Geometry: final body of the model. Coordinates: model frame, mm. Face numbers are marked on the shaded views. Give positions to 0.01 mm unless a question says otherwise; leave off trailing zeros. Write each loop counter-clockwise with the first axis right and the second up, starting at its lowest first coordinate (ties: lowest second). Pieces come first, ordered by that corner, then holes. Notation, with made-up numbers: (70, 87.5) - (126, 87.5) arc R13 ccw to (126, 92.5) - close; hole circle Ø2 at (28.5, 85). An arc over 180 degrees is marked (long way). Use CSV: the item, a comma, the result in double quotes. Start each with the question number.
(1) Section A-A on x = 0. Output: boundary loops of the cut face in (y, z), and give its area (3 significant figures).
(2) Section D-D on z = -3.5. Output: boundary loops of the cut face in (x, y), and give its area (3 significant figures).
(3) Line query: probe 1 along Z at (x, y) = (-21, -23); probe 2 along X at (y, z) = (22, 24.5) (3 decimals); probe 3 along Z at (x, y) = (20.25, 22.75) (3 decimals). Output: solid intervals per line, ascending. Write a range as [from, to].
(4) Section B-B on y = -12. Output: boundary loops of the cut face in (x, z).
(5) Draft query along Y for the marked faces 1, 2 and 3. Return one class per face: released by +Y, released by -Y, zero draft, split by the parting line, or undercut.
(6) First-contact query: pin 1 Ø10 at (x, y) = (9, 6) entering from -Z; pin 2 Ø2.5 at (x, z) = (20.25, -24.5) entering from -Y; pin 3 Ø1.8 at (x, z) = (-20.25, 24.5) entering from +Y; pin 4 Ø5 at (x, y) = (0, 17.5) entering from +Z. Flat tips, straight axial feed; report the tip coordinate or a pass-through.
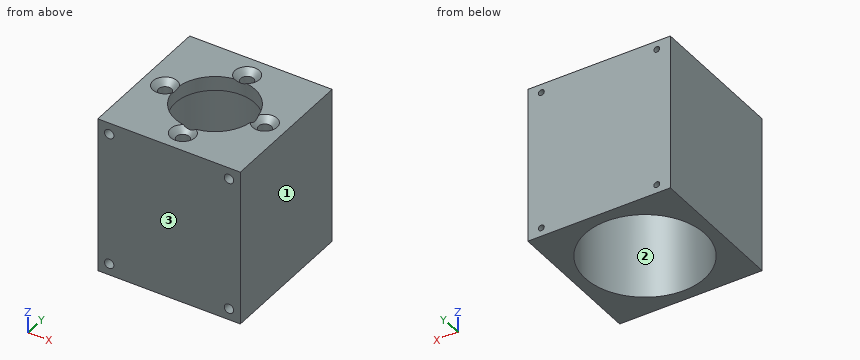
from build123d import *

# Parameters (mm, degrees)
SKETCH_1_W                = 50
SKETCH_1_H                = 50
SKETCH_1_R                = 14
EXTRUDE_2_DEPTH           = 27.5
SKETCH_3_R                = 21
CUT_EXTRUDE_2_DEPTH       = 50
HOLE_WIZARD_M2_5_1_D      = 2.05
HOLE_WIZARD_M2_5_1_DEPTH  = 7.25
HOLE_WIZARD_M2_5_1_TIP    = 0.615882135
HOLE_WIZARD_1_D           = 4.5
HOLE_WIZARD_1_CSINK_D     = 8.6
HOLE_WIZARD_1_CSINK_ANGLE = 90
HOLE_WIZARD_M4_1_D        = 3.3
HOLE_WIZARD_M4_1_DEPTH    = 8.1
HOLE_WIZARD_M4_1_TIP      = 0.991420021


with BuildPart() as part:
    # 草图1 → 凸台-拉伸2 (new, symmetric)
    with BuildSketch(Plane.XY):
        Rectangle(SKETCH_1_W, SKETCH_1_H)
        Circle(SKETCH_1_R, mode=Mode.SUBTRACT)
    extrude(amount=EXTRUDE_2_DEPTH, both=True)

    # 草图3 → 切除-拉伸2 (cut)
    with BuildSketch(Plane(origin=(0, 0, -27.5), x_dir=(-1, 0, 0), z_dir=(0, 0, -1))):
        Circle(SKETCH_3_R)
    extrude(amount=-CUT_EXTRUDE_2_DEPTH, mode=Mode.SUBTRACT)

    # M2.5 螺纹孔1
    with Locations(Plane(origin=(-9.644019955, 25, 9.714634246), x_dir=(1, 0, 0), z_dir=(0, 1, 0))):
        with Locations((29.894019955, 34.214634246), (-10.605980045, -14.785365754), (-10.605980045, 34.214634246), (29.894019955, -14.785365754)):
            Hole(HOLE_WIZARD_M2_5_1_D / 2, depth=HOLE_WIZARD_M2_5_1_DEPTH)
            with Locations((0, 0, -(HOLE_WIZARD_M2_5_1_DEPTH + HOLE_WIZARD_M2_5_1_TIP / 2))):  # 118° drill point
                Cone(0, HOLE_WIZARD_M2_5_1_D / 2, HOLE_WIZARD_M2_5_1_TIP, mode=Mode.SUBTRACT)

    # 打孔尺寸(%根据十字)槽沉头木螺钉的类型1 (through all)
    with Locations(Plane.XY.offset(27.5)):
        with Locations((0, 17.5), (17.5, 0), (0, -17.5), (-17.5, 0)):
            CounterSinkHole(HOLE_WIZARD_1_D / 2, HOLE_WIZARD_1_CSINK_D / 2, counter_sink_angle=HOLE_WIZARD_1_CSINK_ANGLE)

    # M4 螺纹孔1
    with Locations(Plane(origin=(0.5, -25, 0), x_dir=(0, 0, 1), z_dir=(0, -1, 0))):
        with Locations((23.5, 21.5), (-23.5, -20.5), (-23.5, 21.5), (23.5, -20.5)):
            Hole(HOLE_WIZARD_M4_1_D / 2, depth=HOLE_WIZARD_M4_1_DEPTH)
            with Locations((0, 0, -(HOLE_WIZARD_M4_1_DEPTH + HOLE_WIZARD_M4_1_TIP / 2))):  # 118° drill point
                Cone(0, HOLE_WIZARD_M4_1_D / 2, HOLE_WIZARD_M4_1_TIP, mode=Mode.SUBTRACT)


solid = part.part
Check values:
1,outline,"(-25, -27.5) - (-21, -27.5) - (-21, 22.5) - (-19.75, 22.5) - (-19.75, 25.45) - (-21.8, 27.5) - (-25, 27.5) - close; (-15.25, 22.5) - (-14, 22.5) - (-14, 26.7) - (-15.25, 25.45) - close; (14, 22.5) - (15.25, 22.5) - (15.25, 25.45) - (14, 26.7) - close; (19.75, 22.5) - (21, 22.5) - (21, -27.5) - (25, -27.5) - (25, 27.5) - (21.8, 27.5) - (19.75, 25.45) - close"
1,area,"457 mm²"
2,outline,"(-25, -25) - (25, -25) - (25, 25) - (-25, 25) - close; hole circle Ø42 at (0, 0)"
2,area,"1,110 mm²"
3,probe 1,"z = [-27.5, -25.15], [-21.85, 21.85], [25.15, 27.5]"
3,probe 2,"x = [-25, -21.275], [-19.225, 19.225], [21.275, 25]"
3,probe 3,"z = [-27.5, -25.525], [-23.475, 23.475], [25.525, 27.5]"
4,outline,"(-25, -27.5) - (-17.23, -27.5) - (-17.23, 22.5) - (-7.21, 22.5) - (-7.21, 27.5) - (-25, 27.5) - close; (7.21, 22.5) - (17.23, 22.5) - (17.23, -27.5) - (25, -27.5) - (25, 27.5) - (7.21, 27.5) - close"
5,face 1,"zero draft"
5,face 2,"undercut"
5,face 3,"released by -Y"
6,pin 1,"stops at z = 22.5"
6,pin 2,"stops at y = -25"
6,pin 3,"stops at y = 17.67"
6,pin 4,"stops at z = 25.7"
